Can you work these out from the model? Positions are in its coordinate system, mm. Face numbers are marked on the shaded views. A direction names the side the tool comes from. Coordinates: 2 decimals unless noted, no trailing zeros. Loops run counter-clockwise (first coordinate to the right, second up) from the corner with the lowest first, then second, coordinate; pieces in that order, holes last. Notation, with made-up numbers: M 61,47 L 117,47 A16 ccw 117,63 Z; hole C 19.5,-33 d1. An arc over 180 degrees is marked long. Answer as a JSON object with one key per item and string values. Group by question number.
Item 1: Suppose I cut it at B-B (y = 3). Write out the boundary of the cut face in (x, z), then the cut area to 3 significant figures.
Item 2: I'm going to push flat-ended pins straight in: pin 1 Ø19 at (x, y) = (35.5, 20.5) entering from +Z; pin 2 Ø5 at (y, z) = (23, 18) entering from +X; pin 3 Ø4 at (y, z) = (12.5, 16) entering from -X; pin 4 Ø4 at (x, z) = (25, 15) entering from -Y (3 decimals). Where does each tip first touch, or does it pass through?
Item 3: Suppose I cut it at D-D (y = 27). Write out the boundary of the cut face in (x, z).
Item 4: Which directions (+Z, -Z, +X, -X, +Y, -Y) give clear straight access to the entire face, cutting with the end or side of a thin tool? Please do the marked faces 1 and 2.
Item 5: Suppose I cut it at A-A (z = 17.5). Write out the boundary of the cut face in (x, y).
Item 6: If I drill on line 1 (Z direction, x = 26, y = 27); line 2 (X direction, y = 3, z = 18.75); line 3 (Y direction, x = 40.5, z = 22), over which ranges is the centre line in solid material (lowest first)?
Item 7: Suppose I cut it at C-C (x = 33.5). Write out the boundary of the cut face in (y, z), then the cut area to 3 significant figures.
```python
from build123d import *

# Parameters (mm, degrees)
F0_W     = 38.1
F0_H     = 12.7
F1_DEPTH = 50.8
F3_DEPTH = 12.7
F5_DEPTH = 12.7


with BuildPart() as f1:
    # F0 (on Right) → F1 (new body)
    with BuildSketch(Plane.YZ):
        with Locations((19.05, 6.35)):
            Rectangle(F0_W, F0_H)
    extrude(amount=F1_DEPTH)

    # F2 (on face) → F3 (join)
    with BuildSketch(Plane.XY.offset(12.7)):
        Polygon((31.75, 38.1), (0, 38.1), (0, 0), (6.35, 0), align=None)
    extrude(amount=F3_DEPTH)

    # F4 (on face) → F5 (join)
    with BuildSketch(Plane.XY.offset(12.7)):
        Polygon((38.1, 0), (50.8, 0), (50.8, 12.7), align=None)
    extrude(amount=F5_DEPTH)


solid = f1.part
```
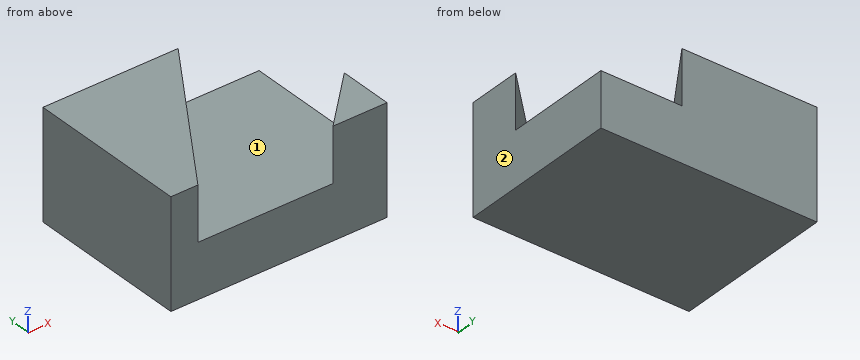
From the geometry:
{
 "1": {"outline": "M 0,0 L 50.8,0 L 50.8,25.4 L 41.1,25.4 L 41.1,12.7 L 8.35,12.7 L 8.35,25.4 L 0,25.4 Z", "area": "874 mm2"},
 "2": {"pin 1": "z = 12.7", "pin 2": "x = 23.35", "pin 3": "x = 0", "pin 4": "y = 24.975"},
 "3": {"outline": "M 0,0 L 50.8,0 L 50.8,12.7 L 24.35,12.7 L 24.35,25.4 L 0,25.4 Z"},
 "4": {"face 1": "+Z", "face 2": "+Z, -Z, +X, +Y, -Y"},
 "5": {"outline": "M 0,0 L 6.35,0 L 31.75,38.1 L 0,38.1 Z; M 38.1,0 L 50.8,0 L 50.8,12.7 Z"},
 "6": {"line 1": "0 to 12.7", "line 2": "0 to 8.35, 41.1 to 50.8", "line 3": "0 to 2.4"},
 "7": {"outline": "M 0,0 L 38.1,0 L 38.1,12.7 L 0,12.7 Z", "area": "484 mm2"}
}
